Can you work these out from the drawing? Everything is in mm from the part's minimum corner. Round coordinates to 2 decimals unless told otherwise and drop trailing zeros. Order: outer loops, then holes, each group sorted by start corner. A loop starts at its lowest first (then second) coordinate and runs counter-clockwise, first axis right, second up. Notation, with made-up numbers: M -27.5,73.25 L -2.5,73.25 A29 cw -2.5,99.25 Z; hole C 25.5,-7 d6. An arc over 180 degrees is marked long. Answer as a JSON object with one key per item and string values. Group by question number.
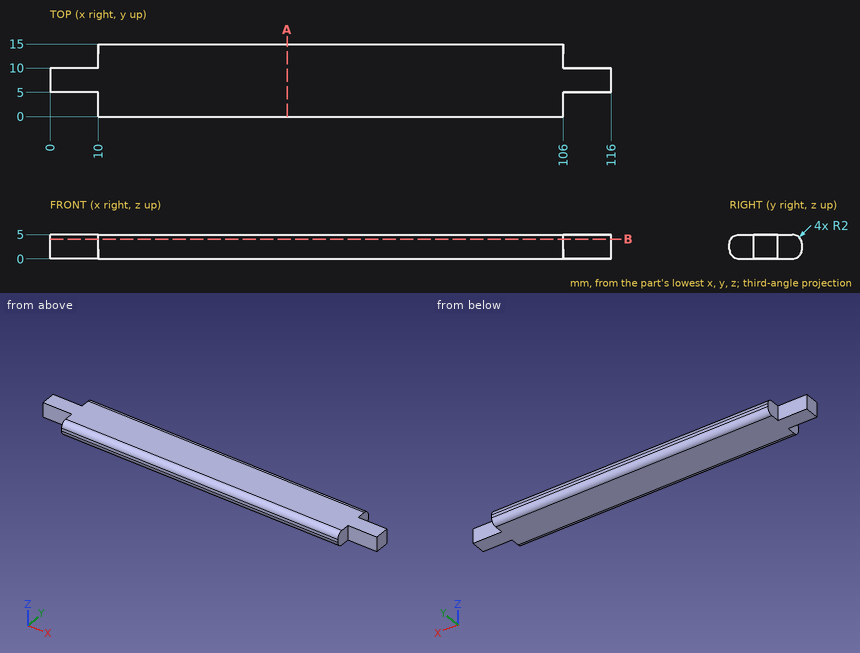
Item 1: I'm going to push flat-ended pins straight in: pin 1 Ø3 at (y, z) = (12, 1.5) entering from +X; pin 2 Ø2.5 at (x, z) = (6, 2) entering from -Y; pin 3 Ø2.5 at (x, z) = (111.5, 2.5) entering from +Y. Where does each tip first touch, or does it pass through?
Item 2: Suppose I cut it at A-A, the plane x = 49. Write out the boundary of the cut face in (y, z), and give its area (3 significant figures).
Item 3: I need wall thicknesses on line 1 (X direction, y = 11.75, z = 4.3); line 2 (Y direction, x = 81.5, z = 1.75); line 3 (Y direction, x = 95.5, z = 4.2). Which ranges of each line are inside material? Lowest first, please.
Item 4: Suppose I cut it at B-B, the plane z = 4.05. Write out the boundary of the cut face in (x, y), and give its area (3 significant figures).
Computed:
{
 "1": {"pin 1": "stops at x = 106", "pin 2": "stops at y = 5", "pin 3": "stops at y = 10"},
 "2": {"outline": "M 0,2 A2 ccw 2,0 L 13,0 A2 ccw 15,2 L 15,3 A2 ccw 13,5 L 2,5 A2 ccw 0,3 Z", "area": "71.6 mm^2"},
 "3": {"line 1": "x = 10 to 106", "line 2": "y = 0.02 to 14.98", "line 3": "y = 0.4 to 14.6"},
 "4": {"outline": "M 0,5 L 10,5 L 10,0.3 L 106,0.3 L 106,5 L 116,5 L 116,10 L 106,10 L 106,14.7 L 10,14.7 L 10,10 L 0,10 Z", "area": "1,480 mm^2"}
}
